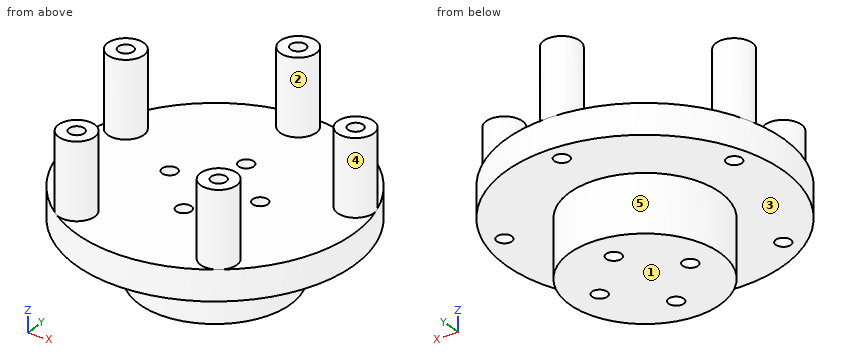
```python
from build123d import *

# Parameters (mm, degrees)
SKETCH1_R           = 23
BOSS_EXTRUDE1_DEPTH = 5
SKETCH2_R           = 3
BOSS_EXTRUDE2_DEPTH = 12.5
SKETCH3_R           = 12.5
BOSS_EXTRUDE3_DEPTH = 9.5
M3_TAPPED_HOLE1_D   = 2.5
CIRPATTERN1_COUNT   = 5
M3_TAPPED_HOLE2_D   = 2.5


with BuildPart() as part:
    # Sketch1 → Boss-Extrude1 (new body)
    with BuildSketch(Plane.XY):
        Circle(SKETCH1_R)
    extrude(amount=BOSS_EXTRUDE1_DEPTH)

    # Sketch2 → Boss-Extrude2 (add)
    with BuildSketch(Plane.XY.offset(5)):
        with Locations(Location((0, 20, 0), (0, 0, 89.999498322))):
            Circle(SKETCH2_R)
        with Locations(Location((19.021130326, 6.180339887, 0), (0, 0, 17.999498258))):
            Circle(SKETCH2_R)
        with Locations(Location((11.755705046, -16.180339887, 0), (0, 0, 305.999498339))):
            Circle(SKETCH2_R)
        with Locations(Location((-11.755705046, -16.180339887, 0), (0, 0, 233.999498303))):
            Circle(SKETCH2_R)
        with Locations(Location((-19.021130326, 6.180339887, 0), (0, 0, 161.999499453))):
            Circle(SKETCH2_R)
    extrude(amount=BOSS_EXTRUDE2_DEPTH)

    # Sketch3 → Boss-Extrude3 (add)
    with BuildSketch(Plane(origin=(0, 0, 0), x_dir=(-1, 0, 0), z_dir=(0, 0, -1))):
        Circle(SKETCH3_R)
    extrude(amount=BOSS_EXTRUDE3_DEPTH)

    # M3 Tapped Hole1 (through all)
    with Locations(Plane.XY.offset(17.5)):
        with Locations((0, 20)):
            m3_tapped_hole1 = Hole(M3_TAPPED_HOLE1_D / 2)

    # CirPattern1: M3 Tapped Hole1 ×5 about axis
    cirpattern1_axis = Axis((0, 0, 0), (0, 0, 1))
    for i in range(1, CIRPATTERN1_COUNT):
        add(m3_tapped_hole1.rotate(cirpattern1_axis, i * 360 / CIRPATTERN1_COUNT), mode=Mode.SUBTRACT)

    # M3 Tapped Hole2 (through all)
    with Locations(Plane(origin=(0, 0, -9.5), x_dir=(-1, 0, 0), z_dir=(0, 0, -1))):
        with Locations((-7.5, 0), (0, 7.5), (7.5, 0), (0, -7.5)):
            Hole(M3_TAPPED_HOLE2_D / 2)


solid = part.part
```
CAD build for the part. Positions are in the model's coordinates, mm. Face numbers are marked on the shaded views. A direction names the side the tool comes from. Round coordinates to 2 decimals unless told otherwise and drop trailing zeros. Write each loop counter-clockwise with the first axis right and the second up, starting at its lowest first coordinate (ties: lowest second). Pieces come first, ordered by that corner, then holes. Notation, with made-up numbers: (77, -39.5) - (102, -39.5) arc R25 ccw to (102, -10.5) - close; hole circle Ø3 at (71, 7.25). An arc over 180 degrees is marked (long way). Write item = value, one per line. Start each with the question number.
Q1. Probe L1, parallel to X at y = 6, z = 16; L2, parallel to X at y = -1, z = -4.5; L3, parallel to Z at x = -6, y = -16. List the from-to ranges inside material, lowest first. Write a range as from..to.
Q2. Band-saw the part on B-B (y = 20). Give the cut face in (x, z).
Q3. Drop flat-ended pins along their axis: pin 1 (1.5 mm diameter, centred on x = 9.5, z = -1, fed in from +Y); pin 2 (2 mm diameter, centred on x = 14.5, y = -9, fed in from -Z); pin 3 (3 mm diameter, centred on x = 16.5, y = -4, fed in from +Z); pin 4 (4 mm diameter, centred on x = 0, y = 7.5, fed in from -Z). Give the stop position or say it passes through.
Q4. Band-saw the part on D-D (x = -4). Give the cut face in (y, z), then the cut area to 3 significant figures.
Q5. Mould opens along X. For the marked faces 3, 4 and 5 say: pulls with the +X half, pulls with the -X half, needs draft (parallel to the pull), parting line crosses it, or undercut.
Q6. Band-saw the part on C-C (x = 7.5). Give the cut face in (y, z).
Q7. Band-saw the part on A-A (z = 6.25). Count the separate pieces of the cut face and the enclosed holes in it, then the cut area to 3 significant figures.
Q8. Which spindle directions (+Z, -Z, +X, -X, +Y, -Y) get a long thin tool onto all of the face, cutting with end or side? Do the marked faces 1 and 2. Say none if no direction does.
Answers below:
q1.L1 = -22.02..-20.26, -17.78..-16.03, 16.03..17.78, 20.26..22.02
q1.L2 = -12.46..-8.25, -6.75..6.75, 8.25..12.46
q1.L3 = 0..5
q2.outline = (-11.36, 0) - (-1.25, 0) - (-1.25, 17.5) - (-3, 17.5) - (-3, 5) - (-11.36, 5) - close; (1.25, 0) - (11.36, 0) - (11.36, 5) - (3, 5) - (3, 17.5) - (1.25, 17.5) - close
q3.pin_1 = 8.93
q3.pin_2 = 0
q3.pin_3 = 5
q3.pin_4 = -9.5
q4.outline = (-22.65, 0) - (-11.84, 0) - (-11.84, -9.5) - (11.84, -9.5) - (11.84, 0) - (22.65, 0) - (22.65, 5) - (-22.65, 5) - close
q4.area = 452 mm2
q5.face_3 = needs draft
q5.face_4 = undercut
q5.face_5 = parting line crosses it
q6.outline = (-21.74, 0) - (-10, 0) - (-10, -9.5) - (-1.25, -9.5) - (-1.25, 5) - (-21.74, 5) - close; (1.25, -9.5) - (10, -9.5) - (10, 0) - (21.74, 0) - (21.74, 5) - (1.25, 5) - close
q7.separate_pieces = 5
q7.enclosed_holes = 5
q7.area = 117 mm2
q8.face_1 = -Z, +X, -X, +Y, -Y
q8.face_2 = +Z
